Print and shaded views of the part. All mm, measured from the part's lowest x, y and z. Give positions to 0.01 mm unless a question says otherwise; leave off trailing zeros. Loops run counter-clockwise (first coordinate to the right, second up) from the corner with the lowest first, then second, coordinate; pieces in that order, holes last. Notation, with made-up numbers: M 22,46.25 L 51,46.25 A31 ccw 51,82.25 Z; hole C -13.5,36.25 d9. An arc over 180 degrees is marked long. Answer in a Markdown table with one row per item.
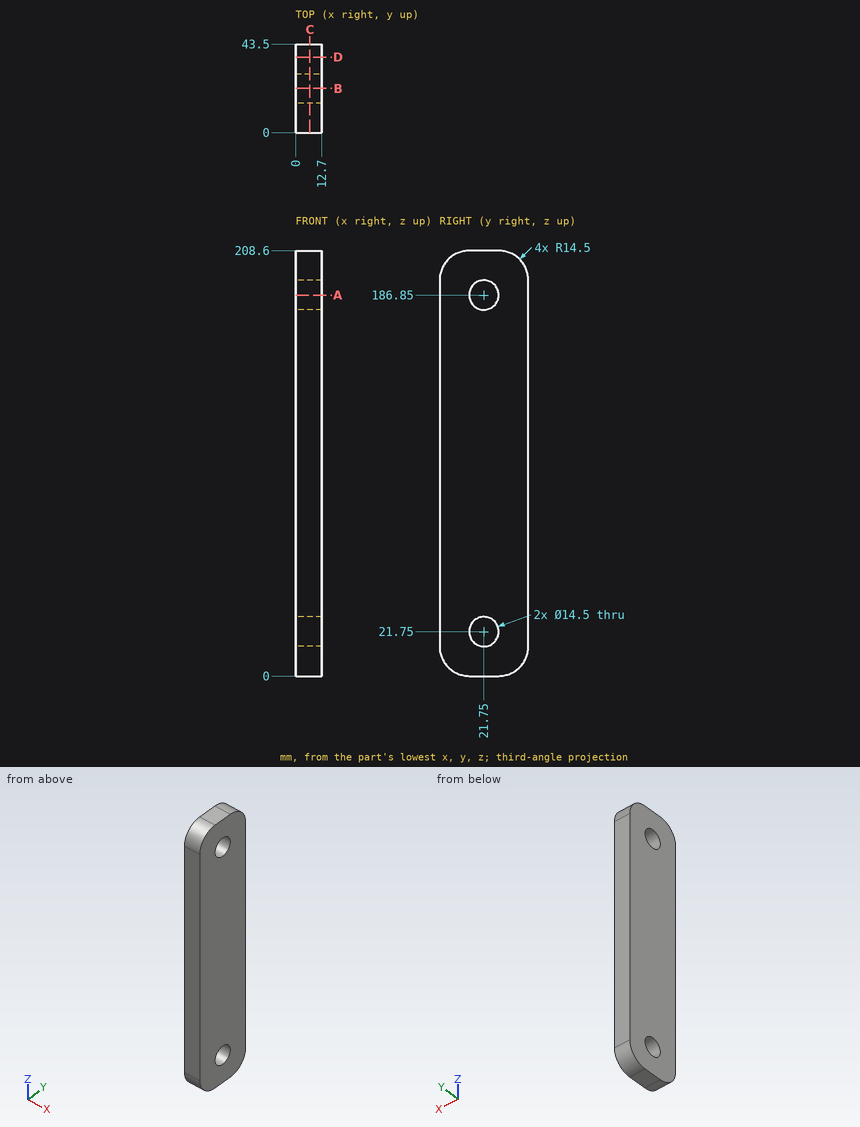
(1) Saw through at A-A, the plane z = 186.85. Give the cut face in (x, y), and give its area (3 significant figures).
Established:
| item | result |
|---|---|
| outline | M 0,0 L 12.7,0 L 12.7,14.5 L 0,14.5 Z; M 0,29 L 12.7,29 L 12.7,43.5 L 0,43.5 Z |
| area | 368 mm2 |
(2) Saw through at C-C, the plane x = 7. Give the cut face in (y, z).
Established:
| item | result |
|---|---|
| outline | M 0,14.5 A14.5 ccw 14.5,0 L 29,0 A14.5 ccw 43.5,14.5 L 43.5,194.1 A14.5 ccw 29,208.6 L 14.5,208.6 A14.5 ccw 0,194.1 Z; hole C 21.75,21.75 d14.5; hole C 21.75,186.85 d14.5 |
(3) Saw through at D-D, the plane y = 37. Give the cut face in (x, z).
Established:
| item | result |
|---|---|
| outline | M 0,2.41 L 12.7,2.41 L 12.7,206.19 L 0,206.19 Z |
(4) Saw through at B-B, the plane y = 21.75. Give the cut face in (x, z), and give its area (3 significant figures).
Established:
| item | result |
|---|---|
| outline | M 0,0 L 12.7,0 L 12.7,14.5 L 0,14.5 Z; M 0,29 L 12.7,29 L 12.7,179.6 L 0,179.6 Z; M 0,194.1 L 12.7,194.1 L 12.7,208.6 L 0,208.6 Z |
| area | 2,280 mm2 |
(5) Flat gauge pin, fed straight in: P1, Ø2, axis at x = 10.5, y = 33, coming from the +Z side. Where does the tip first touch, or does it go through?
Established:
| item | result |
|---|---|
| P1 | stops at z = 208.29 |
(6) Wall check: L1, parallel to Z at x = 4, y = 21.75; L2, parallel to Z at x = 8.25, y = 18; L3, parallel to Z at x = 12.25, y = 6. Give the ranges that are in metal, low to high.
Established:
| item | result |
|---|---|
| L1 | z = 0 to 14.5, 29 to 179.6, 194.1 to 208.6 |
| L2 | z = 0 to 15.55, 27.95 to 180.65, 193.05 to 208.6 |
| L3 | z = 2.75 to 205.85 |
